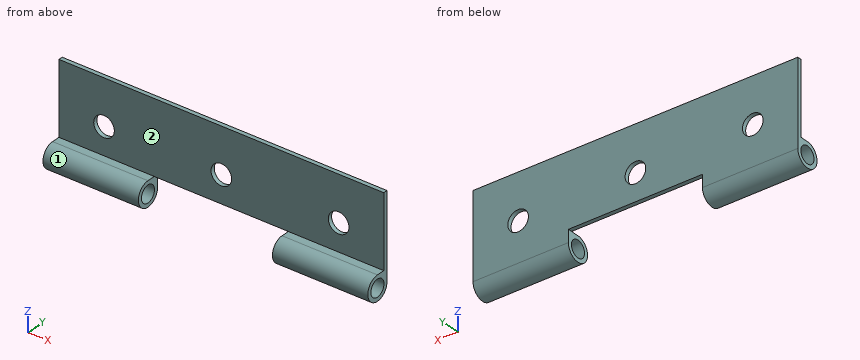
Autodesk Inventor part; units mm, degrees
ref_plane "YZ Plane" through (0, 0, 0) normal (1, 0, 0) x (0, 1, 0)
ref_plane "XZ Plane" through (0, 0, 0) normal (0, 1, 0) x (-1, 0, 0)
ref_plane "XY Plane" through (0, 0, 0) normal (0, 0, 1) x (1, 0, 0)
sketch "Boceto1" plane through (0, 0, 0) normal (0, 1, 0) x (-1, 0, 0)
  line L0 (6.207, 40.007) -> (6.207, 26.007)
  line L1 (6.207, 26.007) -> (-56.793, 26.007)
  line L2 (-56.793, 26.007) -> (-56.793, 40.007)
  line L3 (-56.793, 40.007) -> (6.207, 40.007)
  circle A0 centre (-2.543, 31.257) radius 2
  circle A1 centre (-48.043, 31.257) radius 2
  circle A2 centre (-25.293, 31.257) radius 2
  point P0 (0, 0)
  dimension "d0" = 14
  dimension "d1" = 63
  dimension "d33" = 4
  dimension "d34" = 4
  dimension "d35" = 4
  dimension "d36" = 8.75
  dimension "d37" = 8.75
  dimension "d38" = 8.75
  dimension "d39" = 8.75
  dimension "d40" = 8.75
  dimension "d41" = 31.5
extrude "Extrusión1" add sketch "Boceto1" along normal blind 0.8
sketch "Boceto7" plane through (56.793, 0, 40.007) normal (1, 0, 0) x (0, 0, -1)
  circle A0 centre (16.375, -1.575) radius 2.375
  circle A1 centre (16.375, -1.575) radius 1.625
  line L0 (14, 0) -> (14, 0.8)
  line L1 (0, 0.8) -> (14, 0.8)
  line L2 (0, 0) -> (14, 0)
  line L3 (14, 0) -> (14, -1.575)
  line L4 (14, 0.8) -> (16.375, 0.8)
  line L5 (14, 0.8) -> (14, 0)
  point P0 (40.007, 0)
  dimension "d25" = 4.75
  dimension "d26" = 3.25
extrude "Extrusión4" add sketch "Boceto7" against normal blind 63
sketch "Boceto9" plane through (0, 0.8, 0) normal (0, 1, 0) x (1, 0, 0)
  line L0 (-6.207, -25.257) -> (56.793, -25.257)
  line L1 (-6.207, -40.007) -> (-6.207, -23.632)
  line L2 (12.293, -25.007) -> (12.293, -15.007)
  line L3 (12.293, -15.007) -> (38.2918, -15.007)
  line L4 (38.2918, -15.007) -> (38.2918, -25.257)
  line L5 (38.2918, -25.257) -> (38.2918, -26.007)
  line L6 (56.793, -26.007) -> (-6.207, -26.007)
  line L7 (12.293, -25.007) -> (12.293, -26.007)
  line L8 (12.293, -26.007) -> (38.2918, -26.007)
  line L9 (56.793, -25.257) -> (38.2918, -25.257)
  line L10 (12.293, -25.007) -> (-6.207, -25.007)
  point P0 (0, 0)
  point P1 (38.2918, -25.257)
  point P2 (12.293, -25.257)
  point P3 (38.2918, -25.257)
  dimension "d43" = 26
extrude "Extrusión6" cut sketch "Boceto9" against normal blind 63 contours L7 L2 L3 L4 L0 | L0 L5 L6 L7
properties part number "Ala 1 Bisagra tipo Libro Chica"
For this review, take the finished solid that the model builds, in its own axes (mm). Face numbers are marked on the shaded views. A direction names the side the tool comes from. Give positions to 0.01 mm unless a question says otherwise; leave off trailing zeros. Write each loop counter-clockwise with the first axis right and the second up, starting at its lowest first coordinate (ties: lowest second). Pieces come first, ordered by that corner, then holes. Notation, with made-up numbers: M -22.5,-18.5 L 19.5,-18.5 A20 cw 19.5,5.5 Z; hole C -2,73 d5. An arc over 180 degrees is marked long. Answer as a JSON object with one key per item and string values. Group by question number.
Item 1: For pin 1 Ø6.5 at (x, z) = (25.293, 31.257) entering from -Y; pin 2 Ø0.5 at (x, y) = (47.5, -0.5) entering from +Z; pin 3 Ø3 at (x, z) = (2.543, 31.257) entering from -Y; pin 4 Ø5 at (x, z) = (7.5, 23.5) entering from +Y, all flat-tipped, find the tip position at first contact; note any pin that passes through.
Item 2: Consider section B-B on x = 49. Write out the cut boundary in (y, z) (3 decimals).
Item 3: Consider section D-D on z = 37. Write out the cut boundary in (x, y).
Item 4: Tool access review of the marked faces 1 and 2: name each direction out of +Z, -Z, +X, -X, +Y, -Y from which nothing blocks a thin tool from reaching the whole face with its end or side.
Item 5: Consider section C-C on z = 30. Write out the cut boundary in (x, y), plus the area to 3 significant figures.
Item 6: Consider section A-A on x = 9. Write out the cut boundary in (y, z) (3 decimals).
Item 7: For probe 1 along Y at (x, z) = (19.5, 26.75); probe 2 along Z at (x, y) = (-1, -1.75); probe 3 along Z at (x, y) = (52, -2.3), list the stretches that pass through material, from the lowest coordinate up. Write a range as [from, to].
Check result:
{
 "1": {"pin 1": "stops at y = 0", "pin 2": "stops at z = 26.01", "pin 3": "passes through", "pin 4": "stops at y = 0.8"},
 "2": {"outline": "M -1.575,26.007 A2.375 ccw long 0.8,23.632 L 0.8,29.501 L 0,29.501 L 0,26.007 Z; M 0,33.013 L 0.8,33.013 L 0.8,40.007 L 0,40.007 Z; hole C -1.575,23.632 d3.25"},
 "3": {"outline": "M -6.21,0 L 56.79,0 L 56.79,0.8 L -6.21,0.8 Z"},
 "4": {"face 1": "+X, -X", "face 2": "+Z, +X, -X, -Y"},
 "5": {"outline": "M -6.21,0 L 0.99,0 L 0.99,0.8 L -6.21,0.8 Z; M 4.1,0 L 23.74,0 L 23.74,0.8 L 4.1,0.8 Z; M 26.85,0 L 46.49,0 L 46.49,0.8 L 26.85,0.8 Z; M 49.6,0 L 56.79,0 L 56.79,0.8 L 49.6,0.8 Z", "area": "42.9 mm^2"},
 "6": {"outline": "M -1.575,26.007 A2.375 ccw long 0.8,23.632 L 0.8,40.007 L 0,40.007 L 0,26.007 Z; hole C -1.575,23.632 d3.25"},
 "7": {"probe 1": "y = [0, 0.8]", "probe 2": "z = [21.26, 22.02], [25.25, 26]", "probe 3": "z = [21.37, 22.18], [25.09, 25.89]"}
}
